Design review of the part built by this model. Coordinates are the model's own, in mm. A direction names the side the tool comes from. Coordinates: 2 decimals unless noted, no trailing zeros. Loops run counter-clockwise (first coordinate to the right, second up) from the corner with the lowest first, then second, coordinate; pieces in that order, holes last. Notation, with made-up numbers: (53.25, 60.25) -> (92.25, 60.25) arc R20 cw to (92.25, 96.25) -> close; hole circle Ø1 at (-3, 57). An arc over 180 degrees is marked (long way). Use CSV: the item, a comma, the result in double quotes.
```python
from build123d import *

# Parameters (mm, degrees)
PAD_DEPTH       = 3
SKETCH001_R     = 1.7
HOLE_DEPTH      = 3.001
SKETCH002_W     = 40
SKETCH002_H     = 40
SKETCH002_W_2   = 17
SKETCH002_H_2   = 17
POCKET_DEPTH    = 3.001
SKETCH005_R     = 2.5
PAD001_DEPTH    = 5
SKETCH004_R     = 1.7
HOLE001_DEPTH   = 25
SKETCH003_R     = 5.85
POCKET001_DEPTH = 5


with BuildPart() as part:
    # Sketch → Pad (new body)
    with BuildSketch(Plane.XY):
        with BuildLine():
            Line((10, 130.464466), (10, 13.535534))
            ThreePointArc((10, 13.535534), (11.035534, 11.035534), (13.535534, 10))
            Line((13.535534, 10), (116.464466, 10))
            ThreePointArc((116.464466, 10), (118.964466, 11.035534), (120, 13.535534))
            Line((120, 13.535534), (120, 130.464466))
            ThreePointArc((120, 130.464466), (118.964466, 132.964466), (116.464466, 134))
            Line((116.464466, 134), (13.535534, 134))
            ThreePointArc((13.535534, 134), (11.035534, 132.964466), (10, 130.464466))
        make_face()
    extrude(amount=PAD_DEPTH)

    # Sketch001 → Hole (cut, through all)
    with BuildSketch(Plane.XY):
        with Locations((15, 129)):
            Circle(SKETCH001_R)
        with Locations((15, 79)):
            Circle(SKETCH001_R)
        with Locations((15, 15)):
            Circle(SKETCH001_R)
        with Locations((115, 15)):
            Circle(SKETCH001_R)
        with Locations((115, 65)):
            Circle(SKETCH001_R)
        with Locations((115, 129)):
            Circle(SKETCH001_R)
    extrude(amount=HOLE_DEPTH, mode=Mode.SUBTRACT)

    # Sketch002 → Pocket (cut, through all)
    with BuildSketch(Plane.XY):
        with Locations((65, 70)):
            Rectangle(SKETCH002_W, SKETCH002_H)
        with Locations((65.5, 23.5)):
            Rectangle(SKETCH002_W_2, SKETCH002_H_2)
    extrude(amount=POCKET_DEPTH, mode=Mode.SUBTRACT)

    # Sketch005 → Pad001 (join)
    with BuildSketch(Plane.XY):
        with Locations((90, 56)):
            Circle(SKETCH005_R)
        with Locations((111, 56)):
            Circle(SKETCH005_R)
        with Locations((90, 25)):
            Circle(SKETCH005_R)
        with Locations((111, 25)):
            Circle(SKETCH005_R)
    extrude(amount=-PAD001_DEPTH)

    # Sketch004 → Hole001 (cut)
    with BuildSketch(Plane.XY):
        with Locations((90, 56)):
            Circle(SKETCH004_R)
        with Locations((111, 56)):
            Circle(SKETCH004_R)
        with Locations((90, 25)):
            Circle(SKETCH004_R)
        with Locations((111, 25)):
            Circle(SKETCH004_R)
    extrude(amount=-HOLE001_DEPTH, mode=Mode.SUBTRACT)

    # Sketch003 → Pocket001 (cut)
    with BuildSketch(Plane.XY):
        with Locations((37, 24)):
            Circle(SKETCH003_R)
    extrude(amount=POCKET001_DEPTH, mode=Mode.SUBTRACT)


solid = part.part
```
Item 1: Clearance check with flat-ended pins moving along their axes: pin 1 (2.5 mm diameter, centred on x = 90, y = 25.5, fed in from -Z); pin 2 (2 mm diameter, centred on x = 102, y = 99.5, fed in from -Z); pin 3 (2.5 mm diameter, centred on x = 15, y = 79, fed in from -Z). State where each tip first meets the part, or that it passes through.
Checked values:
pin 1,"z = -5"
pin 2,"z = 0"
pin 3,"through"
Item 2: Draft analysis for pull direction X (two halves, no side actions). For faces 1 (the face through (11.06, 132.99, 1.48)), 2 (the face through (92, 55, -5)), 3 (the face through (88.16, 26.69, -2.46)), 4 (the face through (109.3, 25.07, -2.46)), state which applies: pulls with the +X half, pulls with the -X half, needs draft (parallel to the pull), parting line crosses it, or undercut.
Checked values:
face 1,"pulls with the -X half"
face 2,"needs draft"
face 3,"undercut"
face 4,"undercut"
Item 3: Add section B-B (x = 81). Give the boundary of the cut face in (y, z).
Checked values:
outline,"(10, 0) -> (50, 0) -> (50, 3) -> (10, 3) -> close; (90, 0) -> (134, 0) -> (134, 3) -> (90, 3) -> close"
Item 4: Add section D-D (y = 129). Give the boundary of the cut face in (x, z).
Checked values:
outline,"(10, 0) -> (13.3, 0) -> (13.3, 3) -> (10, 3) -> close; (16.7, 0) -> (113.3, 0) -> (113.3, 3) -> (16.7, 3) -> close; (116.7, 0) -> (120, 0) -> (120, 3) -> (116.7, 3) -> close"
Item 5: Add section A-A (y = 56). Give the boundary of the cut face in (x, z).
Checked values:
outline,"(10, 0) -> (45, 0) -> (45, 3) -> (10, 3) -> close; (85, 0) -> (87.5, 0) -> (87.5, -5) -> (88.3, -5) -> (88.3, 0) -> (91.7, 0) -> (91.7, -5) -> (92.5, -5) -> (92.5, 0) -> (108.5, 0) -> (108.5, -5) -> (109.3, -5) -> (109.3, 0) -> (112.7, 0) -> (112.7, -5) -> (113.5, -5) -> (113.5, 0) -> (120, 0) -> (120, 3) -> (85, 3) -> close"
Item 6: Machinability: for faces 5 (the face through (65, 32, 1)), 6 (the face through (118.99, 132.94, 1.48)), 7 (the face through (111, 56, 0)), which of the approach directions +Z, -Z, +X, -X, +Y, -Y give a long, thin tool a straight path to every point of the face, cutting with its end or side? Answer none if there is none.
Checked values:
face 5,"+Z, -Z"
face 6,"+Z, -Z, +X, +Y"
face 7,"-Z"
Item 7: To check wall thickness, follow line 1 along Y through (x, z) = (15, 0.7); line 2 along X through (y, z) = (129, 0.8); line 3 along Y through (x, z) = (64.5, 0.75). State the ranges of each line that lie inside material, in increasing order.
Checked values:
line 1,"10 to 13.3, 16.7 to 77.3, 80.7 to 127.3, 130.7 to 134"
line 2,"10 to 13.3, 16.7 to 113.3, 116.7 to 120"
line 3,"10 to 15, 32 to 50, 90 to 134"
Item 8: Add section C-C (z = -1.25). Give the boundary of the cut face in (x, y).
Checked values:
outline,"circle Ø5 at (90, 25); circle Ø5 at (90, 56); circle Ø5 at (111, 25); circle Ø5 at (111, 56); hole circle Ø3.4 at (90, 25); hole circle Ø3.4 at (90, 56); hole circle Ø3.4 at (111, 25); hole circle Ø3.4 at (111, 56)"
